Verification items for the finished model (mm, model axes). A direction names the side the tool comes from. Give positions to 0.01 mm unless a question says otherwise; leave off trailing zeros. Loops run counter-clockwise (first coordinate to the right, second up) from the corner with the lowest first, then second, coordinate; pieces in that order, holes last. Notation, with made-up numbers: (-23.75, -5.5) - (19.25, -5.5) arc R34 cw to (19.25, 28.5) - close; hole circle Ø7 at (20, 11). An arc over 180 degrees is marked (long way). One line per item, written item: value. Start each with the question number.
1. Mould release check, pull along Y, two halves, no side actions. Record for faces 1 (the flat face through (-42.5, -7, 4)), 2 (the flat face through (-19, 0, 2)), 3 (the cylindrical face through (2.465, -26.577, 21.429)): pulls with the +Y half, pulls with the -Y half, needs draft (parallel to the pull), parting line crosses it, or undercut.
2. Scan lines: L1, parallel to Z at x = 2.05, y = -27.5; L2, parallel to Z at x = -4, y = -20. Record each from-to range of solid material in increasing order. Write a range as [from, to].
3. Gauge pin test, flat ends, axial feed: pin 1 (8 mm diameter, centred on x = -14.5, y = -12, fed in from +Z); pin 2 (4 mm diameter, centred on x = -23.5, z = 9.5, fed in from -Y); pin 3 (2 mm diameter, centred on x = -30, y = -21.5, fed in from +Z). Record the tip position at first contact, or that the pin passes through.
4. Sectioned sample at B-B (z = 2.75). Record the cut outline in (x, y), plus the area to 3 significant figures.
5. Sectioned sample at A-A (y = -27.5). Record the cut outline in (x, z), plus the area to 3 significant figures.
6. Access from +Z, -Z, +X, -X, +Y, -Y to the whole of each face (thin tool, end or side, straight path). Record for faces 4 (the flat face through (-18, -28, 0)), 5 (the flat face through (-20, -27, 5)), 6 (the flat face through (5, -28, 12)), 7 (the flat face through (-40, -27, 2)), 8 (the flat face through (-21, -8, 8.183)).
7. Sectioned sample at D-D (y = -22). Record the cut outline in (x, z), plus the area to 3 significant figures.
8. Sectioned sample at C-C (x = -1.5). Record the cut outline in (y, z), plus the area to 3 significant figures.
from build123d import *

# Parameters (mm, degrees)
F0_W     = 40
F0_H     = 5
F1_DEPTH = 55
F2_R     = 2
F3_DEPTH = 5
F5_DEPTH = 42.5


with BuildPart() as f1:
    # F0 (on Front) → F1 (new body)
    with BuildSketch(Plane.XZ):
        with Locations((-20, 2.5)):
            Rectangle(F0_W, F0_H)
    extrude(amount=F1_DEPTH)

    # F2 (on Right) → F3 (join)
    with BuildSketch(Plane.YZ):
        Polygon((-5.740549, 0), (0, 0), (0, 4.96355), (-55, 4.96355), (-55, 0), align=None)
        with BuildLine():
            Line((-55, 4.96355), (0, 4.96355))
            Line((0, 4.96355), (-22.910616, 27.806423))
            ThreePointArc((-22.910616, 27.806423), (-27.5, 29.703428), (-32.089384, 27.806423))
            Line((-32.089384, 27.806423), (-55, 4.96355))
        make_face()
        with Locations((-27.5, 23.203428)):
            Circle(F2_R, mode=Mode.SUBTRACT)
    extrude(amount=F3_DEPTH)

    # F4 (on Right) → F5 (join)
    with BuildSketch(Plane.YZ):
        Polygon((-55, 5), (-55, 0), (-41.870234, 0), (-41.870234, 8.235325), (-51.870234, 8.235325), align=None)
        Polygon((0, 0), (0, 5), (-3.183106, 8.18286), (-13.183106, 8.18286), (-13.183106, 0), align=None)
    extrude(amount=-F5_DEPTH)


solid = f1.part
Results are:
1. face 1: needs draft
1. face 2: pulls with the +Y half
1. face 3: undercut
2. L1: z = [0, 21.2], [25.2, 29.7]
2. L2: z = [0, 5]
3. pin 1: stops at z = 8.18
3. pin 2: stops at y = -52.58
3. pin 3: stops at z = 5
4. outline: (-42.5, -55) - (5, -55) - (5, 0) - (-42.5, 0) - (-42.5, -13.18) - (-40, -13.18) - (-40, -41.87) - (-42.5, -41.87) - close
4. area: 2,540 mm^2
5. outline: (-40, 0) - (5, 0) - (5, 21.2) - (0, 21.2) - (0, 5) - (-40, 5) - close; (0, 25.2) - (5, 25.2) - (5, 29.7) - (0, 29.7) - close
5. area: 329 mm^2
6. face 4: -Z, +X, -X, +Y, -Y
6. face 5: +Z, -X
6. face 6: +Z, -Z, +X, +Y, -Y
6. face 7: +Z, -Z, -X
6. face 8: +Z, -X, +Y
7. outline: (-40, 0) - (5, 0) - (5, 26.9) - (0, 26.9) - (0, 5) - (-40, 5) - close
7. area: 334 mm^2
8. outline: (-55, 0) - (0, 0) - (0, 5) - (-3.18, 8.18) - (-13.18, 8.18) - (-13.18, 5) - (-41.87, 5) - (-41.87, 8.24) - (-51.87, 8.24) - (-55, 5) - close
8. area: 349 mm^2
